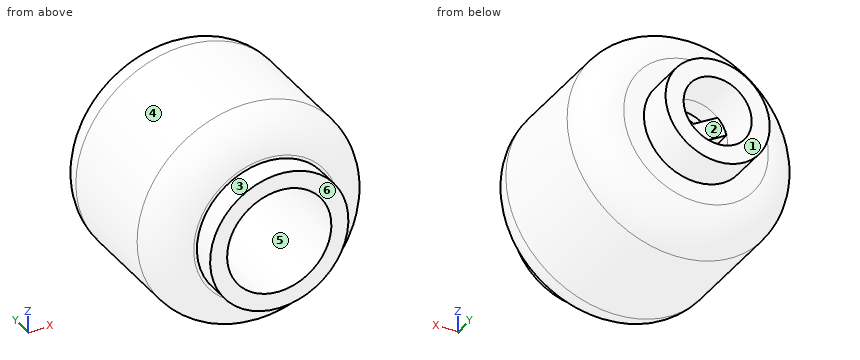
```python
from build123d import *

# Parameters (mm, degrees)
AIR_HOLE_DEPTH    = 10
CIRCPATTERN_COUNT = 3


with BuildPart() as part:
    # Sketch1 → Head Revolve (revolve)
    with BuildSketch(Plane(origin=(0, 0, 0), x_dir=(0, 0, -1), z_dir=(1, 0, 0))):
        with BuildLine():
            Line((0, 8.5), (0, 9.4))
            Line((0, 9.4), (1.6, 9.4))
            Line((1.6, 9.4), (1.6, 11.4))
            Line((1.6, 11.4), (2.45, 11.4))
            Line((2.45, 11.4), (2.45, 9.6))
            Line((2.45, 9.6), (3.4, 9.6))
            ThreePointArc((3.4, 9.6), (4.602081528, 9.102081528), (5.1, 7.9))
            Line((5.1, 7.9), (5.1, 2.8))
            ThreePointArc((5.1, 2.8), (4.602081528, 1.597918472), (3.4, 1.1))
            Line((3.4, 1.1), (3.25, 1.1))
            Line((3.25, 1.1), (3.25, 0))
            Line((3.25, 0), (2.45, 0))
            Line((2.45, 0), (2.45, 8.5))
            Line((2.45, 8.5), (0, 8.5))
        make_face()
    revolve(axis=Axis((0, 16.31372549, 0), (0, -1, 0)))

    # Sketch2 → Air Hole (cut)
    with BuildSketch(Plane(origin=(0, 9.4, 0), x_dir=(1, 0, 0), z_dir=(0, 1, 0))):
        with BuildLine():
            Line((-0.42, 1.543891188), (-0.42, 0.242487113))
            Line((-0.42, 0.242487113), (-1.547048989, -0.408214924))
            ThreePointArc((-1.547048989, -0.408214924), (-1.385640646, 0.8), (-0.42, 1.543891188))
        make_face()
    air_hole = extrude(amount=-AIR_HOLE_DEPTH, mode=Mode.SUBTRACT)

    # CircPattern: Air Hole ×3 about axis
    circpattern_axis = Axis((0, 0, 0), (0, 1, 0))
    for i in range(1, CIRCPATTERN_COUNT):
        add(air_hole.rotate(circpattern_axis, i * 360 / CIRCPATTERN_COUNT), mode=Mode.SUBTRACT)


solid = part.part
```
The model under review builds one solid part; all positions refer to its coordinate system, in mm. Face numbers are marked on the shaded views. A direction names the side the tool comes from. Round coordinates to 2 decimals unless told otherwise and drop trailing zeros. Loops run counter-clockwise (first coordinate to the right, second up) from the corner with the lowest first, then second, coordinate; pieces in that order, holes last. Notation, with made-up numbers: M 66.25,10.5 L 73.25,10.5 A20 cw 73.25,19.5 Z; hole C 81,47 d4. An arc over 180 degrees is marked long. Answer as a JSON object with one key per item and string values.
(1) Tool access review of the marked faces 1, 2 and 3: name each direction out of +Z, -Z, +X, -X, +Y, -Y from which nothing blocks a thin tool from reaching the whole face with its end or side.
Resolved:
{"face 1": "+Z, -Z, +X, -X, +Y", "face 2": "+Y", "face 3": "-Y"}
(2) Take a section at A-A on z = 0. Give the boundary of the cut face in (x, y).
Resolved:
{"outline": "M -5.1,2.8 A1.7 ccw -3.4,1.1 L -3.25,1.1 L -3.25,0 L -2.45,0 L -2.45,8.5 L -1.6,8.5 L -1.6,11.4 L -2.45,11.4 L -2.45,9.6 L -3.4,9.6 A1.7 ccw -5.1,7.9 Z; M -0.84,8.5 L 0.84,8.5 L 0.84,9.4 L -0.84,9.4 Z; M 1.6,8.5 L 2.45,8.5 L 2.45,0 L 3.25,0 L 3.25,1.1 L 3.4,1.1 A1.7 ccw 5.1,2.8 L 5.1,7.9 A1.7 ccw 3.4,9.6 L 2.45,9.6 L 2.45,11.4 L 1.6,11.4 Z"}
(3) Clearance check with flat-ended pins moving along their axes: P1, Ø3, axis at y = 6.5, z = 2.5, coming from the +X side; P2, Ø1.9, axis at x = 0, z = 0, coming from the -Y side; P3, Ø1, axis at y = 9, z = -1, coming from the -X side. State where each tip first meets the part, or that it passes through.
Resolved:
{"P1": "x = 5", "P2": "y = 8.5", "P3": "x = -4.91"}
(4) Draft analysis for pull direction Z (two halves, no side actions). For the marked faces 4, 5 and 6, state which applies: released by +Z, released by -Z, zero draft, split by the parting line, or undercut.
Resolved:
{"face 4": "split by the parting line", "face 5": "undercut", "face 6": "zero draft"}
(5) Take a section at B-B on y = 3.5. Give the boundary of the cut face in (x, z).
Resolved:
{"outline": "C 0,0 d10.2; hole C 0,0 d4.9"}
(6) To check wall thickness, follow line 1 along X through (y, z) = (4.5, 0); line 2 along X through (y, z) = (10.6, 0); line 3 along Y through (x, z) = (3.5, -0.25). State the ranges of each line that lie inside material, in increasing order.
Resolved:
{"line 1": "-5.1 to -2.45, 2.45 to 5.1", "line 2": "-2.45 to -1.6, 1.6 to 2.45", "line 3": "1.1 to 9.6"}
(7) Take a section at C-C on y = 1.75. Give the boundary of the cut face in (x, z), and give its area (3 significant figures).
Resolved:
{"outline": "C 0,0 d9.47; hole C 0,0 d4.9", "area": "51.6 mm²"}
